Input: dimensioned drawing with shaded views. Units: mm. Origin: part minimum x, y, z. A direction names the side the tool comes from. Give positions to 0.01 mm unless a question says otherwise; leave off trailing zeros. Loops run counter-clockwise (first coordinate to the right, second up) from the corner with the lowest first, then second, coordinate; pieces in that order, holes last. Notation, with made-up numbers: (22.25, -39.75) -> (58.25, -39.75) arc R25 cw to (58.25, -25.75) -> close; hole circle Ø5 at (-28.75, 34.5). An arc over 180 degrees is marked (long way). Answer as a JSON object with one key per item and string values.
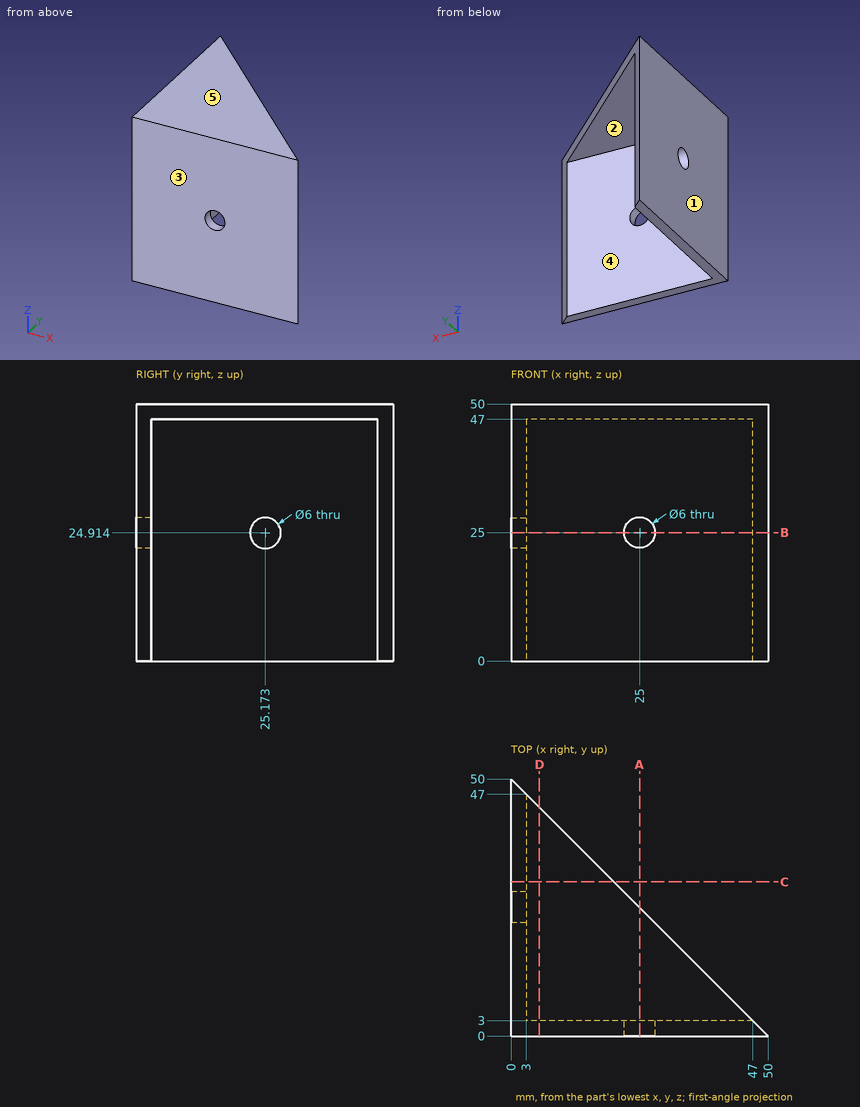
Q1. Pin query (flat end, axial travel): pin 1 (3 mm diameter, centred on y = 23.5, z = 43.5, fed in from +X); pin 2 (6 mm diameter, centred on x = 11.5, y = 7, fed in from -Z); pin 3 (4 mm diameter, centred on x = 17.5, z = 7, fed in from +Y). Return the tip coordinate at first contact, or that it passes through.
Evaluation:
{"pin 1": "stops at x = 3", "pin 2": "stops at z = 47", "pin 3": "stops at y = 3"}
Q2. Section B-B, the plane z = 25. Return the cut outline in (x, y), then the cut area to 3 significant figures.
Evaluation:
{"outline": "(0, 0) -> (22, 0) -> (22, 3) -> (3, 3) -> (3, 22.17) -> (0, 22.17) -> close; (0, 28.17) -> (3, 28.17) -> (3, 47) -> (0, 50) -> close; (28, 0) -> (50, 0) -> (47, 3) -> (28, 3) -> close", "area": "246 mm2"}
Q3. Draft query along Y for the marked faces 3, 4 and 5. Return one class per face: +Y half, -Y half, draft (parallel to the pull), parting line (faces both ways), or undercut.
Evaluation:
{"face 3": "-Y half", "face 4": "+Y half", "face 5": "draft"}
Q4. Ray query, line 1 along X through (y, z) = (24.5, 46.5); line 2 along Z through (x, y) = (25, 0.9). Return the intervals inside material, ascending.
Evaluation:
{"line 1": "x = 0 to 3", "line 2": "z = 0 to 22, 28 to 50"}
Q5. Section C-C, the plane y = 30. Return the cut outline in (x, z).
Evaluation:
{"outline": "(0, 0) -> (3, 0) -> (3, 47) -> (20, 47) -> (20, 50) -> (0, 50) -> close"}
Q6. Section A-A, the plane x = 25. Return the cut outline in (y, z), then the cut area to 3 significant figures.
Evaluation:
{"outline": "(0, 0) -> (3, 0) -> (3, 22) -> (0, 22) -> close; (0, 28) -> (3, 28) -> (3, 47) -> (25, 47) -> (25, 50) -> (0, 50) -> close", "area": "198 mm2"}
Q7. Access query for the marked faces 1 and 2. Directions: +Z, -Z, +X, -X, +Y, -Y. A direction counts if a zero-diameter tool reaches every point of the face in a straight line with its end or side. Return the directions, or none.
Evaluation:
{"face 1": "+Z, -Z, -X, +Y, -Y", "face 2": "-Z, +X, +Y"}
Q8. Section D-D, the plane x = 5.5. Return the cut outline in (y, z).
Evaluation:
{"outline": "(0, 0) -> (3, 0) -> (3, 47) -> (44.5, 47) -> (44.5, 50) -> (0, 50) -> close"}
